Verification items for the finished model (mm, model axes). Give positions to 0.01 mm unless a question says otherwise; leave off trailing zeros.
(1) Gauge pin test, flat end, axial feed: pin 1 (0.9 mm diameter, centred on x = -4.5, y = 0, fed in from +Z). Record the tip position at first contact, or that the pin passes through.
(2) Scan lines: L1, parallel to Y at x = 0, z = 0.5; L2, parallel to Y at x = -33, z = 1; L3, parallel to X at y = 5, z = 1.95. Record each from-to range of solid material in increasing order.
(3) Sectioned sample at A-A on z = 1.4. Count the separate pieces of the cut face and the enclosed holes in it, plus the area to 3 significant figures.
Autodesk Inventor part; units mm, degrees
ref_plane "YZ Plane" through (0, 0, 0) normal (1, 0, 0) x (0, 1, 0)
ref_plane "XZ Plane" through (0, 0, 0) normal (0, 1, 0) x (-1, 0, 0)
ref_plane "XY Plane" through (0, 0, 0) normal (0, 0, 1) x (1, 0, 0)
sketch "Boceto1" plane through (0, 0, 0) normal (0, 0, 1) x (1, 0, 0)
  line L0 (-45, -14.5) -> (45, -14.5)
  line L1 (45, -14.5) -> (45, 14.5)
  line L2 (45, 14.5) -> (-45, 14.5)
  line L3 (-45, 14.5) -> (-45, -14.5)
  line L4 (45, -14.5) -> (-45, 14.5) construction
  circle A0 centre (0, 0) radius 2
  line L5 (0, 0) -> (4.5, 0) construction
  line L6 (0, 0) -> (4.5, 0)
  circle A1 centre (0, 4.5) radius 0.75
  circle A2 centre (4.5, 0) radius 0.75
  circle A3 centre (0, -4.5) radius 0.75
  circle A4 centre (-4.5, 0) radius 0.75
  circle A5 centre (-42, 0) radius 0.75
  circle A6 centre (-37.5, 0) radius 2
  circle A7 centre (-33, 0) radius 0.75
  circle A8 centre (-37.5, 4.5) radius 0.75
  circle A9 centre (-37.5, -4.5) radius 0.75
  circle A10 centre (37.5, 0) radius 2
  circle A11 centre (42, 0) radius 0.75
  circle A12 centre (37.5, 4.5) radius 0.75
  circle A13 centre (33, 0) radius 0.75
  circle A14 centre (37.5, -4.5) radius 0.75
  dimension "d0" = 90
  dimension "d1" = 29
  dimension "d2" = 4
  dimension "d8" = 1.5
  dimension "d9" = 1.5
  dimension "d10" = 1.5
  dimension "d11" = 1.5
  dimension "d23" = 4
  dimension "d25" = 1.5
  dimension "d28" = 1.5
  dimension "d29" = 1.5
  dimension "d35" = 4
  dimension "d36" = 1.5
  dimension "d37" = 1.5
  dimension "d38" = 1.5
  dimension "d39" = 1.5
extrude "Extrusión1" add sketch "Boceto1" along normal blind 2
properties part number "frontal2" material "Acero, galvanizado"
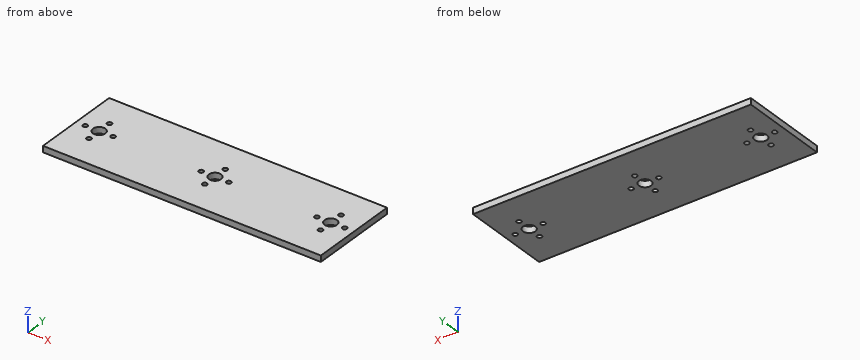
Ans:
1. pin 1: passes through
2. L1: y = -14.5 to -5.25, -3.75 to -2, 2 to 3.75, 5.25 to 14.5
2. L2: y = -14.5 to -0.75, 0.75 to 14.5
2. L3: x = -45 to -38.06, -36.94 to -0.56, 0.56 to 36.94, 38.06 to 45
3. separate pieces: 1
3. enclosed holes: 15
3. area: 2,550 mm2
